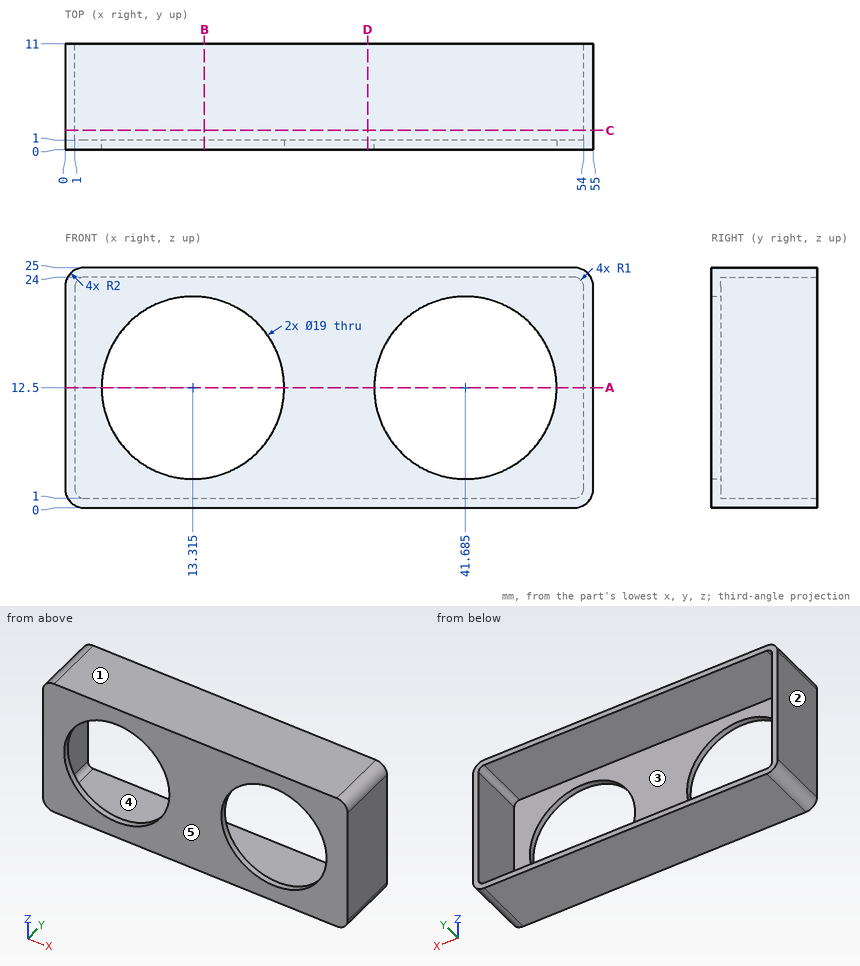
The figure shows three views and two pictorial views of one solid part (mm, origin at its lowest corner). Answer the questions. A direction names the side the tool comes from. Coordinates: 2 decimals unless noted, no trailing zeros. Order: outer loops, then holes, each group sorted by start corner. A loop starts at its lowest first (then second) coordinate and runs counter-clockwise, first axis right, second up.
Q1. A cutting plane is placed at D-D, the plane x = 31.5. Write down the section's boundary in (y, z).
Q2. Which of the six approach directions +Z, -Z, +X, -X, +Y, -Y give full straight-line access (tool end or side, diameter ignored) to the marked faces 4 and 5?
Q3. A cutting plane is placed at B-B, the plane x = 14.5. Write down the section's boundary in (y, z).
Q4. A cutting plane is placed at A-A, the plane z = 12.5. Write down the section's boundary in (x, y) (1 decimal), and give its area (3 significant figures).
Q5. Given P1, Ø11.5, axis at x = 41.68, z = 12.5, coming from the -Y side; P2, Ø1, axis at x = 22, z = 8.5, coming from the +Y side, each flat-ended and moving along its own axis, determine where each tip first touches the part or whether it passes through.
Q6. For a pull along Z with two mould halves and no side action, classify the marked faces 1, 2 and 3 as pulls with the +Z half, pulls with the -Z half, needs draft (parallel to the pull), parting line crosses it, or undercut.
Q7. A cutting plane is placed at C-C, the plane y = 2. Write down the section's boundary in (x, z).
Q8. Consider line 1 (Z direction, x = 11.5, y = 4.75); line 2 (X direction, y = 10.25, z = 17.25); line 3 (Y direction, x = 35, z = 3). Determine where each line is inside the solid, lowest interval first.
Answers follow:
1. outline: (0, 0) - (11, 0) - (11, 1) - (1, 1) - (1, 24) - (11, 24) - (11, 25) - (0, 25) - close
2. face 4: +Y
2. face 5: +Z, -Z, +X, -X, -Y
3. outline: (0, 0) - (11, 0) - (11, 1) - (1, 1) - (1, 3.07) - (0, 3.07) - close; (0, 21.93) - (1, 21.93) - (1, 24) - (11, 24) - (11, 25) - (0, 25) - close
4. outline: (0, 0) - (3.8, 0) - (3.8, 1) - (1, 1) - (1, 11) - (0, 11) - close; (22.8, 0) - (32.2, 0) - (32.2, 1) - (22.8, 1) - close; (51.2, 0) - (55, 0) - (55, 11) - (54, 11) - (54, 1) - (51.2, 1) - close
4. area: 37.0 mm2
5. P1: passes through
5. P2: stops at y = 1
6. face 1: pulls with the +Z half
6. face 2: needs draft
6. face 3: undercut
7. outline: (0, 2) arc R2 ccw to (2, 0) - (53, 0) arc R2 ccw to (55, 2) - (55, 23) arc R2 ccw to (53, 25) - (2, 25) arc R2 ccw to (0, 23) - close; hole (1, 2) arc R1 ccw to (2, 1) - (53, 1) arc R1 ccw to (54, 2) - (54, 23) arc R1 ccw to (53, 24) - (2, 24) arc R1 ccw to (1, 23) - close
8. line 1: z = 0 to 1, 24 to 25
8. line 2: x = 0 to 1, 54 to 55
8. line 3: y = 0 to 1
